Answer from the drawing. Dimensions are ordinates in mm from the lowest x, y and z of the part. Round coordinates to 2 decimals unless told otherwise and drop trailing zeros. Write each loop counter-clockwise with the first axis right and the second up, starting at its lowest first coordinate (ties: lowest second). Pieces come first, ordered by that corner, then holes. Notation, with made-up numbers: (71, 75) -> (122, 75) arc R27 ccw to (122, 99) -> close; hole circle Ø9 at (77, 81). An arc over 180 degrees is marked (long way). Return JSON: item names as keys, results as strings. Group by question number.
(1) A cutting plane is placed at C-C on y = 7.25. Give the vertices of the cut face in (x, z).
(2) A cutting plane is placed at A-A on x = 41.3. Give the vertices of the cut face in (y, z).
(3) The mould has two halves that part along Z. Classify the marked faces 1, 2 and 3: released by +Z, released by -Z, zero draft, split by the parting line, or undercut.
(4) A cutting plane is placed at B-B on y = 3. Give the vertices of the cut face in (x, z).
(5) Straight lines are drawn through the part: line 1 (X direction, y = 12.4, z = 41.3); line 2 (X direction, y = 11.25, z = 75) (1 decimal); line 3 (Z direction, x = 33.5, y = 11). For each, find the intervals that lie inside material, in ascending order.
(6) Given pin 1 (1.5 mm diameter, centred on y = 9.5, z = 15, fed in from +X); pin 2 (4 mm diameter, centred on x = 41.3, z = 5.8, fed in from -Y); pin 3 (6 mm diameter, centred on x = 52.5, y = 4, fed in from -Z) (1 decimal); pin 4 (2.5 mm diameter, centred on x = 5.8, z = 41.3, fed in from +Y), each flat-ended and moving along its own axis, determine where each tip first touches the part or whether it passes through.
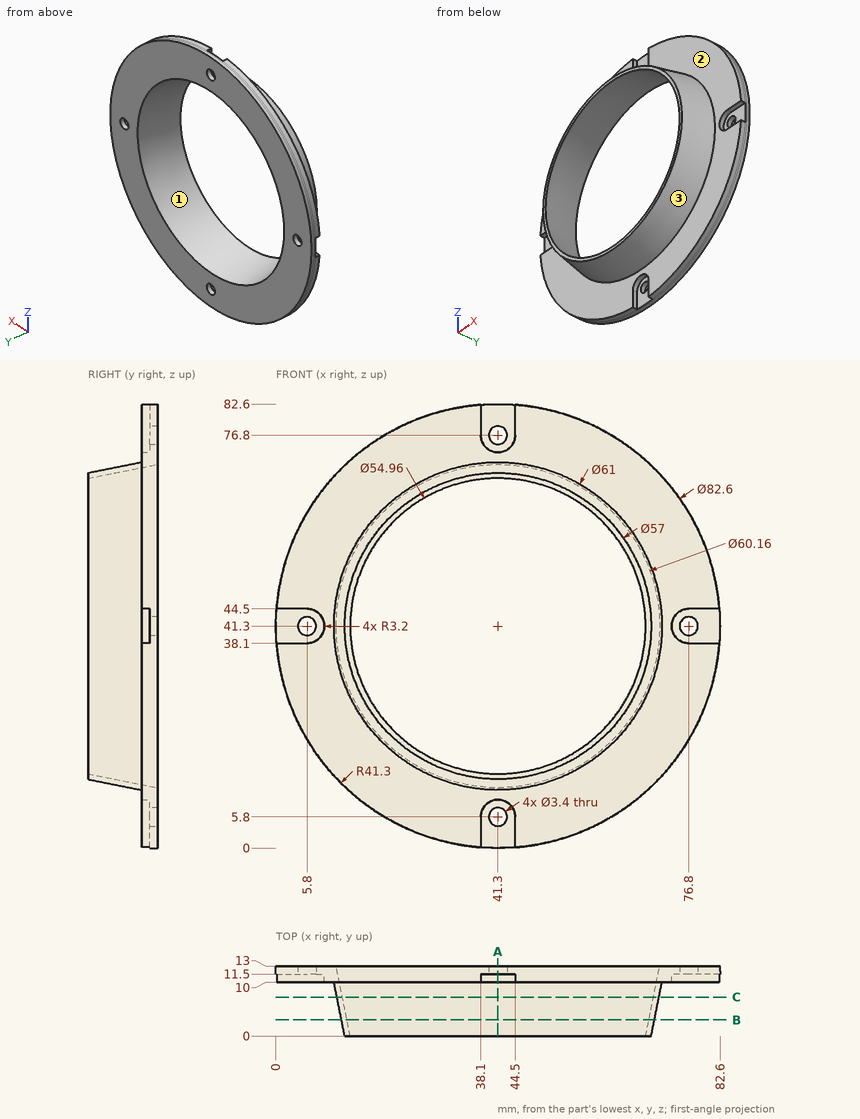
Checks:
{
 "1": {"outline": "circle Ø59.9 at (41.3, 41.3); hole circle Ø57.86 at (41.3, 41.3)"},
 "2": {"outline": "(0, 12.8) -> (10, 10.8) -> (10, 9) -> (11.5, 9) -> (11.5, 7.5) -> (13, 7.5) -> (13, 11.22) -> (0, 13.82) -> close; (0, 68.78) -> (13, 71.38) -> (13, 75.1) -> (11.5, 75.1) -> (11.5, 73.6) -> (10, 73.6) -> (10, 71.8) -> (0, 69.8) -> close; (11.5, 0) -> (13, 0) -> (13, 4.1) -> (11.5, 4.1) -> close; (11.5, 78.5) -> (13, 78.5) -> (13, 82.6) -> (11.5, 82.6) -> close"},
 "3": {"face 1": "undercut", "face 2": "zero draft", "face 3": "split by the parting line"},
 "4": {"outline": "circle Ø58.2 at (41.3, 41.3); hole circle Ø56.16 at (41.3, 41.3)"},
 "5": {"line 1": "x = 0 to 4.1, 7.5 to 11.34, 71.26 to 75.1, 78.5 to 82.6", "line 2": "x = 17.4 to 38.7, 43.9 to 65.2", "line 3": "z = 0.74 to 12.66, 69.94 to 81.86"},
 "6": {"pin 1": "stops at x = 73.6", "pin 2": "stops at y = 11.5", "pin 3": "stops at z = 13", "pin 4": "passes through"}
}
